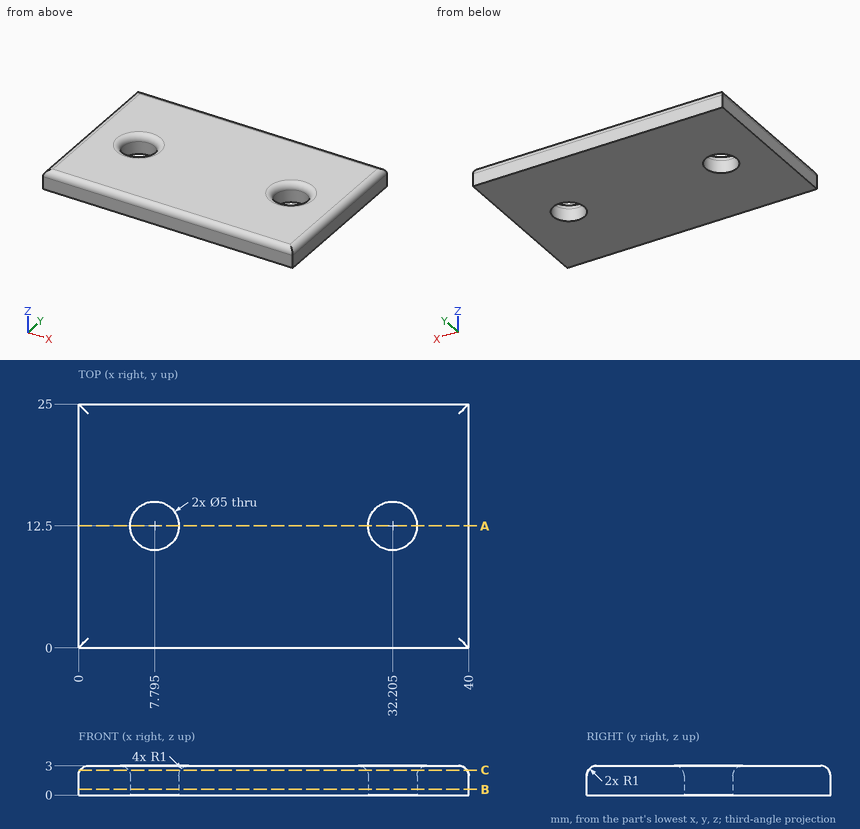
Check sheet for the drawn part. Datum: minimum x, y, z corner. Units: mm. Give positions to 0.01 mm unless a question says otherwise; leave off trailing zeros. Write each loop counter-clockwise with the first axis right and the second up, starting at its lowest first coordinate (ties: lowest second). Pieces come first, ordered by that corner, then holes. Notation, with made-up numbers: M 43.5,39.5 L 57.5,39.5 A19 ccw 57.5,58.5 Z; hole C 11.5,14.25 d10. An arc over 180 degrees is marked long. Write item = value, one per line.
(1) Sectioned sample at B-B (z = 0.6). Record the cut outline in (x, y) (3 decimals), then the cut area to 3 significant figures.
Found:
outline = M 0,0 L 40,0 L 40,25 L 0,25 Z; hole C 7.795,12.5 d5; hole C 32.205,12.5 d5
area = 961 mm2
(2) Sectioned sample at A-A (y = 12.5). Record the cut outline in (x, z) (3 decimals), then the cut area to 3 significant figures.
Found:
outline = M 0,0 L 5.295,0 L 5.295,2 A1 ccw 4.295,3 L 1,3 A1 ccw 0,2 Z; M 10.295,0 L 29.705,0 L 29.705,2 A1 ccw 28.705,3 L 11.295,3 A1 ccw 10.295,2 Z; M 34.705,0 L 40,0 L 40,2 A1 ccw 39,3 L 35.705,3 A1 ccw 34.705,2 Z
area = 88.7 mm2
(3) Go/stop test with a flat-tipped pin: pin 1 Ø3 at (x, y) = (7.795, 12.5) entering from -Z (3 decimals). Record where the tip stops, or that it passes through.
Found:
pin_1 = through
(4) Sectioned sample at C-C (z = 2.55). Record the cut outline in (x, y) (3 decimals).
Found:
outline = M 0.165,0.165 L 39.835,0.165 L 39.835,24.835 L 0.165,24.835 Z; hole C 7.795,12.5 d5.33; hole C 32.205,12.5 d5.33
(5) Material ranges on line 1 (X direction, y = 13.5, z = 1.2); line 2 (X direction, y = 13.75, z = 2.55); line 3 (Y direction, x = 8.5, z = 2.35), recorded low to high.
Found:
line_1 = 0 to 5.5, 10.09 to 29.91, 34.5 to 40
line_2 = 0.16 to 5.44, 10.15 to 29.85, 34.56 to 39.84
line_3 = 0.06 to 10.04, 14.96 to 24.94
